Can you work these out from the model? Positions are in its coordinate system, mm. A direction names the side the tool comes from. Round coordinates to 2 decimals unless told otherwise and drop trailing zeros. Order: outer loops, then holes, each group sorted by start corner. A loop starts at its lowest first (then second) coordinate and runs counter-clockwise, first axis right, second up. Notation, with made-up numbers: M 28,62.5 L 84,62.5 A13 cw 84,79.5 Z; hole C 24,6.25 d11. An arc over 180 degrees is marked long. Answer as a JSON object with one key per item and string values. Group by question number.
from build123d import *

# Parameters (mm, degrees)
F0_W     = 203.2
F0_H     = 19.05
F1_DEPTH = 558.8
F2_R     = 19.05
F2_W     = 12.7
F2_H     = 12.7
F3_DEPTH = 25.4


with BuildPart() as f1:
    # F0 (on Front) → F1 (new body)
    with BuildSketch(Plane.XZ):
        Rectangle(F0_W, F0_H)
    extrude(amount=F1_DEPTH)

    # F2 (on face) → F3 (cut)
    with BuildSketch(Plane.XY.offset(9.525)):
        with Locations((-63.5, -101.6)):
            Circle(F2_R)
        with Locations((63.5, -101.6)):
            Circle(F2_R)
        with Locations((-63.5, -419.1)):
            Circle(F2_R)
        with Locations((63.5, -419.1)):
            Circle(F2_R)
        with Locations((-63.5, -6.35)):
            Rectangle(F2_W, F2_H)
    extrude(amount=-F3_DEPTH, mode=Mode.SUBTRACT)


solid = f1.part
Item 1: Suppose I cut it at B-B, the plane y = -101.6. Write out the boundary of the cut face in (x, z) (3 decimals), and give its area (3 significant figures).
Item 2: On a 3-axis mill with a long thin cutter (end or side, diameter ignored), from which of +Z, -Z, +X, -X, +Y, -Y can I reach the whole of each face in a straight line? I mean faces 4 (the face through (-1, -275, 9.525)), 5 (the face through (-64, -12.7, 0)). Say none if no direction works.
Item 3: Suppose I cut it at A-A, the plane z = 5.25. Write out the boundary of the cut face in (x, y).
Item 4: Suppose I cut it at C-C, the plane x = 63.5. Write out the boundary of the cut face in (y, z) (3 decimals), and give its area (3 significant figures).
Item 5: If we mould it in two halves opening along X, with no side actions, what happens to faces 1 (the face through (-101.6, -275, 0)), 2 (the face through (101.6, -275, 0)), 3 (the face through (-65.98, -400.212, 0.133))? For each: +X half, -X half, draft (parallel to the pull), parting line (faces both ways), or undercut.
Item 6: I need wall thicknesses on line 1 (Y direction, x = -63.5, z = -0.5); line 2 (Y direction, x = 63.5, z = -1.5); line 3 (X direction, y = -119, z = 2). Which ranges of each line are inside material? Lowest first, please.
Item 7: I'm going to push a flat-ended pin straight in: pin 1 Ø23 at (x, y) = (-63.5, -419.1) entering from +Z (3 decimals). Where does the tip first touch, or does it pass through?
Computed:
{
 "1": {"outline": "M -101.6,-9.525 L -82.55,-9.525 L -82.55,9.525 L -101.6,9.525 Z; M -44.45,-9.525 L 44.45,-9.525 L 44.45,9.525 L -44.45,9.525 Z; M 82.55,-9.525 L 101.6,-9.525 L 101.6,9.525 L 82.55,9.525 Z", "area": "2,420 mm^2"},
 "2": {"face 4": "+Z, +X, -X, +Y, -Y", "face 5": "+Z, -Z, +Y"},
 "3": {"outline": "M -101.6,-558.8 L 101.6,-558.8 L 101.6,0 L -57.15,0 L -57.15,-12.7 L -69.85,-12.7 L -69.85,0 L -101.6,0 Z; hole C -63.5,-419.1 d38.1; hole C -63.5,-101.6 d38.1; hole C 63.5,-419.1 d38.1; hole C 63.5,-101.6 d38.1"},
 "4": {"outline": "M -558.8,-9.525 L -438.15,-9.525 L -438.15,9.525 L -558.8,9.525 Z; M -400.05,-9.525 L -120.65,-9.525 L -120.65,9.525 L -400.05,9.525 Z; M -82.55,-9.525 L 0,-9.525 L 0,9.525 L -82.55,9.525 Z", "area": "9,190 mm^2"},
 "5": {"face 1": "-X half", "face 2": "+X half", "face 3": "undercut"},
 "6": {"line 1": "y = -558.8 to -438.15, -400.05 to -120.65, -82.55 to -12.7", "line 2": "y = -558.8 to -438.15, -400.05 to -120.65, -82.55 to 0", "line 3": "x = -101.6 to -71.26, -55.74 to 55.74, 71.26 to 101.6"},
 "7": {"pin 1": "passes through"}
}
